from build123d import *

# Parameters (mm, degrees)
SKETCH1_R           = 12.5
SKETCH1_R_2         = 6
BOSS_EXTRUDE2_DEPTH = 7.5
BOSS_EXTRUDE3_DEPTH = 4.5


with BuildPart() as part:
    # Sketch1 → Boss-Extrude2 (new body, symmetric)
    with BuildSketch(Plane.XY):
        with BuildLine():
            Line((2.01059306, -9.376516335), (2.01059306, 58.959050431))
            ThreePointArc((2.01059306, 58.959050431), (-2.28940694, 79.038194443), (-6.58940694, 58.959050431))
            Line((-6.58940694, 58.959050431), (-6.58940694, -9.376516335))
            ThreePointArc((-6.58940694, -9.376516335), (-2.28940694, -53.961805557), (2.01059306, -9.376516335))
        make_face()
        with Locations((-2.28940694, -31.461805557)):
            Circle(SKETCH1_R, mode=Mode.SUBTRACT)
        with Locations((-2.28940694, 68.538194443)):
            Circle(SKETCH1_R_2, mode=Mode.SUBTRACT)
        with BuildLine():
            Line((-4.58940694, 56.760673481), (-4.58940694, -7.572268098))
            ThreePointArc((-4.58940694, -7.572268098), (-2.28940694, -7.461805557), (0.01059306, -7.572268098))
            Line((0.01059306, -7.572268098), (0.01059306, 56.760673481))
            ThreePointArc((0.01059306, 56.760673481), (-2.28940694, 56.538194443), (-4.58940694, 56.760673481))
        make_face(mode=Mode.SUBTRACT)
    extrude(amount=BOSS_EXTRUDE2_DEPTH, both=True)

    # Sketch2 → Boss-Extrude3 (add, symmetric)
    with BuildSketch(Plane.XY):
        with BuildLine():
            Line((-4.58940694, 56.760673481), (-4.58940694, -7.572268098))
            ThreePointArc((-4.58940694, -7.572268098), (-2.28940694, -7.461805557), (0.01059306, -7.572268098))
            Line((0.01059306, -7.572268098), (0.01059306, 56.760673481))
            ThreePointArc((0.01059306, 56.760673481), (-2.28940694, 56.538194443), (-4.58940694, 56.760673481))
        make_face()
    extrude(amount=BOSS_EXTRUDE3_DEPTH, both=True)


solid = part.part
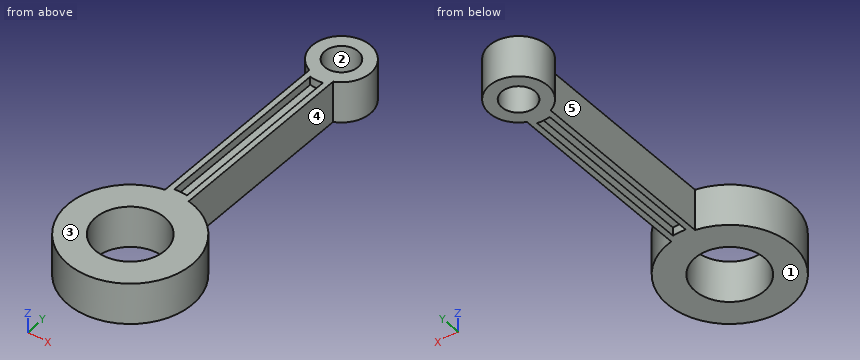
Source: CAD feature listing. Evaluate the final solid. Frame: model axes, mm. Face numbers are marked on the shaded views. A direction names the side the tool comes from. Coordinates: 2 decimals unless noted, no trailing zeros. Loops run counter-clockwise (first coordinate to the right, second up) from the corner with the lowest first, then second, coordinate; pieces in that order, holes last. Notation, with made-up numbers: M 74,63.5 L 79,63.5 A16 cw 79,82.5 Z; hole C -10.75,-3 d9. An arc over 180 degrees is marked long. Answer in a Markdown table with one row per item.
Q1. Section A-A on y = -34.5. Return the cut outline in (x, z), plus the area to 3 significant figures.
Answers below:
| item | result |
|---|---|
| outline | M -24.58,-7.5 L -14.41,-7.5 L -14.41,7.5 L -24.58,7.5 Z; M 9.84,-7.5 L 20,-7.5 L 20,7.5 L 9.84,7.5 Z |
| area | 305 mm^2 |
Q2. First-contact query: pin 1 (2 mm diameter, centred on x = 7.5, z = -4.5, fed in from +Y); pin 2 (6 mm diameter, centred on y = 19, z = -0.5, fed in from -X); pin 3 (1.5 mm diameter, centred on y = 30.5, z = 6.5, fed in from +X); pin 4 (6 mm diameter, centred on x = -10.5, y = -28, fed in from -Z). Flat tips, straight axial feed; report the tip coordinate or a pass-through.
Answers below:
| item | result |
|---|---|
| pin 1 | stops at y = 74.28 |
| pin 2 | stops at x = -6.59 |
| pin 3 | stops at x = 2.01 |
| pin 4 | passes through |
Q3. Draft query along Y for the marked faces 1 and 2. Return one class per face: pulls with the +Y half, pulls with the -Y half, needs draft (parallel to the pull), parting line crosses it, or undercut.
Answers below:
| item | result |
|---|---|
| face 1 | needs draft |
| face 2 | undercut |
Q4. Section D-D on z = -2.25. Return the cut outline in (x, y).
Answers below:
| item | result |
|---|---|
| outline | M -6.59,-9.38 A22.5 ccw long 2.01,-9.38 L 2.01,58.96 A10.5 ccw long -6.59,58.96 Z; hole C -2.29,-31.46 d25; hole C -2.29,68.54 d12 |
Q5. Section C-C on y = 17. Return the cut outline in (x, z), plus the area to 3 significant figures.
Answers below:
| item | result |
|---|---|
| outline | M -6.59,-7.5 L -4.59,-7.5 L -4.59,-4.5 L 0.01,-4.5 L 0.01,-7.5 L 2.01,-7.5 L 2.01,7.5 L 0.01,7.5 L 0.01,4.5 L -4.59,4.5 L -4.59,7.5 L -6.59,7.5 Z |
| area | 101 mm^2 |
Q6. Set-up query: the marked faces 3, 4 and 5. Return all of +Z, -Z, +X, -X, +Y, -Y with unobstructed straight access to the full face (end or side cutting, diameter ignored); none if empty.
Answers below:
| item | result |
|---|---|
| face 3 | +Z, +X, -X, +Y, -Y |
| face 4 | +Z, -Z, +X |
| face 5 | +Z, -Z, -X |
Q7. Section B-B on x = -1.5. Return the cut outline in (y, z).
Answers below:
| item | result |
|---|---|
| outline | M -53.95,-7.5 L -43.94,-7.5 L -43.94,7.5 L -53.95,7.5 Z; M -18.99,-7.5 L -7.47,-7.5 L -7.47,-4.5 L 56.56,-4.5 L 56.56,-7.5 L 62.59,-7.5 L 62.59,7.5 L 56.56,7.5 L 56.56,4.5 L -7.47,4.5 L -7.47,7.5 L -18.99,7.5 Z; M 74.49,-7.5 L 79.01,-7.5 L 79.01,7.5 L 74.49,7.5 Z |
Q8. Ray query, probe 1 along Y at (x, z) = (-5.5, 0); probe 2 along Y at (x, z) = (0, 4.25); probe 3 along X at (y, z) = (28, -6.25). Return the intervals inside material, ascending. Write a range as from..to.
Answers below:
| item | result |
|---|---|
| probe 1 | y = -53.73..-43.54, -19.38..63.47, 73.61..78.54 |
| probe 2 | y = -53.85..-43.75, -19.17..62.99, 74.08..78.79 |
| probe 3 | x = -6.59..-4.59, 0.01..2.01 |
